Could you check a few things on this model? Use its own coordinates, in mm. A direction names the side the tool comes from. Coordinates: 2 decimals unless noted, no trailing zeros. Write each loop counter-clockwise with the first axis right and the second up, starting at its lowest first coordinate (ties: lowest second). Pieces come first, ordered by that corner, then holes.
```python
from build123d import *

# Parameters (mm, degrees)
SKETCH1_W            = 15
SKETCH1_H            = 50
BOSS_EXTRUDE1_DEPTH  = 10
SKETCH2_W            = 3
SKETCH2_H            = 15
CUT_EXTRUDE1_DEPTH   = 20
SKETCH3_R            = 1.5
CUT_EXTRUDE2_DEPTH   = 20
SKETCH4_W            = 5
SKETCH4_H            = 15
CUT_EXTRUDE3_DEPTH   = 20
CUT_EXTRUDE4_REACH   = 32.943
SKETCH5_R            = 1.5
FILLET1_R            = 2
SKETCH6_W            = 5
SKETCH6_H            = 10
BOSS_EXTRUDE2_DEPTH  = 149.4
FILLET1_OF_MIRROR5_R = 2
FILLET2_R            = 5


with BuildPart() as part:
    # Sketch1 → Boss-Extrude1 (new body)
    with BuildSketch(Plane.XY):
        with Locations((-8.26142132, 1.154822335)):
            Rectangle(SKETCH1_W, SKETCH1_H)
    boss_extrude1 = extrude(amount=BOSS_EXTRUDE1_DEPTH)

    # Sketch2 → Cut-Extrude1 (cut)
    with BuildSketch(Plane(origin=(-0.76142132, 0, 0), x_dir=(0, 0, -1), z_dir=(1, 0, 0))):
        with Locations((-1.5, 18.654822335)):
            Rectangle(SKETCH2_W, SKETCH2_H)
        with Locations((-8.5, 18.654822335)):
            Rectangle(SKETCH2_W, SKETCH2_H)
    cut_extrude1 = extrude(amount=-CUT_EXTRUDE1_DEPTH, mode=Mode.SUBTRACT)

    # Sketch3 → Cut-Extrude2 (cut)
    with BuildSketch(Plane(origin=(0, 0, 3), x_dir=(-1, 0, 0), z_dir=(0, 0, -1))):
        with Locations(Location((4.26142132, 16.154822335, 0), (0, 0, 90))):
            Circle(SKETCH3_R)
        with Locations(Location((12.26142132, 16.154822335, 0), (0, 0, 90))):
            Circle(SKETCH3_R)
    cut_extrude2 = extrude(amount=-CUT_EXTRUDE2_DEPTH, mode=Mode.SUBTRACT)

    # Sketch4 → Cut-Extrude3 (cut)
    with BuildSketch(Plane(origin=(-0.76142132, 0, 0), x_dir=(0, 0, -1), z_dir=(1, 0, 0))):
        with Locations((-7.5, -16.345177665)):
            Rectangle(SKETCH4_W, SKETCH4_H)
    cut_extrude3 = extrude(amount=-CUT_EXTRUDE3_DEPTH, mode=Mode.SUBTRACT)

    # Sketch5 → Cut-Extrude4 (cut, up to next)
    with BuildSketch(Plane.XY.offset(5), mode=Mode.PRIVATE) as cut_extrude4_sk1:
        with Locations((-8.26142132, -16.345177665)):
            Circle(SKETCH5_R)
    cut_extrude4_tool1 = extrude(cut_extrude4_sk1.sketch, amount=-CUT_EXTRUDE4_REACH, mode=Mode.PRIVATE) & part.part
    cut_extrude4 = cut_extrude4_tool1.solids().sort_by_distance((-8.261421, -16.345178, 5))[0]
    add(cut_extrude4, mode=Mode.SUBTRACT)

    # Fillet1
    fillet1_edges = [part.edges().sort_by_distance(p)[0] for p in [
        (-8.26142132, 11.154822335, 3),
        (-8.26142132, 11.154822335, 7),
        (-8.26142132, -8.845177665, 5),
    ]]
    fillet(fillet1_edges, radius=FILLET1_R)

    # Sketch6 → Boss-Extrude2 (add)
    with BuildSketch(Plane.ZY.offset(15.76142132)):
        with Locations((2.5, -18.845177665)):
            Rectangle(SKETCH6_W, SKETCH6_H)
    extrude(amount=BOSS_EXTRUDE2_DEPTH)

    # Mirror5: Boss-Extrude1, Cut-Extrude1, Cut-Extrude2, Cut-Extrude3, Cut-Extrude4 across plane
    add(boss_extrude1.mirror(Plane.ZY.offset(90.46142132)))
    add(cut_extrude1.mirror(Plane.ZY.offset(90.46142132)), mode=Mode.SUBTRACT)
    add(cut_extrude2.mirror(Plane.ZY.offset(90.46142132)), mode=Mode.SUBTRACT)
    add(cut_extrude3.mirror(Plane.ZY.offset(90.46142132)), mode=Mode.SUBTRACT)
    add(cut_extrude4.mirror(Plane.ZY.offset(90.46142132)), mode=Mode.SUBTRACT)

    # Fillet1 of Mirror5
    fillet1_of_mirror5_edges = [part.edges().sort_by_distance(p)[0] for p in [
        (-172.66142132, 11.154822335, 3),
        (-172.66142132, 11.154822335, 7),
        (-172.66142132, -8.845177665, 5),
    ]]
    fillet(fillet1_of_mirror5_edges, radius=FILLET1_OF_MIRROR5_R)

    # Fillet2
    fillet2_edges = [part.edges().sort_by_distance(p)[0] for p in [
        (-180.16142132, -23.845177665, 2.5),
        (-0.76142132, -23.845177665, 2.5),
        (-165.16142132, -13.845177665, 2.5),
        (-15.76142132, -13.845177665, 2.5),
    ]]
    fillet(fillet2_edges, radius=FILLET2_R - 0.0001)  # a hair under: the kernel refuses the full size


solid = part.part
```
1. For pin 1 (3.5 mm diameter, centred on x = -12.26, y = 16.15, fed in from -Z); pin 2 (5 mm diameter, centred on x = -140, z = 4.5, fed in from +Y); pin 3 (5 mm diameter, centred on x = -151.5, z = 9, fed in from -Y); pin 4 (14.5 mm diameter, centred on x = -121, y = -17, fed in from +Z), each with a flat end and sliding along its axis, tell me the tip position at first contact or that it passes through.
Verdict:
pin 1: stops at z = 3
pin 2: stops at y = -13.85
pin 3: passes through
pin 4: stops at z = 5
2. I want a section at A-A on y = 8. Please give me the cut outline in (x, z).
Verdict:
outline: (-180.16, 0) - (-165.16, 0) - (-165.16, 10) - (-180.16, 10) - close; (-15.76, 0) - (-0.76, 0) - (-0.76, 10) - (-15.76, 10) - close
3. I want a section at B-B on x = -34.5. Please give me the cut outline in (y, z).
Verdict:
outline: (-23.85, 0) - (-13.85, 0) - (-13.85, 5) - (-23.85, 5) - close
4. If we mould it in two halves opening along X, with no side actions, what happens to faces 6 (the face through (-0.761, 3, 5)), 7 (the face through (-8, -8.845, 9)), 8 (the face through (-175.197, 15.83, 4.972))? For each: pulls with the +X half, pulls with the -X half, needs draft (parallel to the pull), parting line crosses it, or undercut.
Verdict:
face 6: pulls with the +X half
face 7: needs draft
face 8: undercut
5. Please list where these lines run through material, in increasing order: line 1 along X through (y, z) = (-6, 2.75); line 2 along Y through (x, z) = (-112, 1.5); line 3 along Z through (x, y) = (-116, -19.5).
Verdict:
line 1: x = -180.16 to -165.16, -15.76 to -0.76
line 2: y = -23.85 to -13.85
line 3: z = 0 to 5
6. On a 3-axis mill with a long thin cutter (end or side, diameter ignored), from which of +Z, -Z, +X, -X, +Y, -Y can I reach the whole of each face in a straight line? I mean faces 1 (the face through (-180.161, 3, 5)), 2 (the face through (-15.761, 5, 5)), 3 (the face through (-173, 20, 7)), 4 (the face through (-8, 20, 3)), 5 (the face through (-12.84, 17.54, 4.97)). Say none if no direction works.
Verdict:
face 1: +Z, -Z, -X, +Y, -Y
face 2: +Z, -Z, +Y
face 3: +Z, +X, -X, +Y
face 4: -Z, +X, -X, +Y
face 5: +Z, -Z
